```python
from build123d import *

# Parameters (mm, degrees)
SKETCH1_W           = 620
SKETCH1_H           = 130
SKETCH1_R           = 10
SKETCH1_W_2         = 18
SKETCH1_H_2         = 50
SKETCH1_W_3         = 37.615580966
SKETCH1_H_3         = 15.499548612
BOSS_EXTRUDE1_DEPTH = 18


with BuildPart() as part:
    # Sketch1 → Boss-Extrude1 (new body)
    with BuildSketch(Plane.XY):
        with Locations((310, -65)):
            Rectangle(SKETCH1_W, SKETCH1_H)
        with Locations((310, -65)):
            Circle(SKETCH1_R, mode=Mode.SUBTRACT)
        with Locations((22.856274172, -65)):
            Rectangle(SKETCH1_W_2, SKETCH1_H_2, mode=Mode.SUBTRACT)
        with Locations((310, -104.250225694)):
            Rectangle(SKETCH1_W_3, SKETCH1_H_3, mode=Mode.SUBTRACT)
        with Locations((597.143725828, -65)):
            Rectangle(SKETCH1_W_2, SKETCH1_H_2, mode=Mode.SUBTRACT)
    extrude(amount=BOSS_EXTRUDE1_DEPTH)


solid = part.part
```
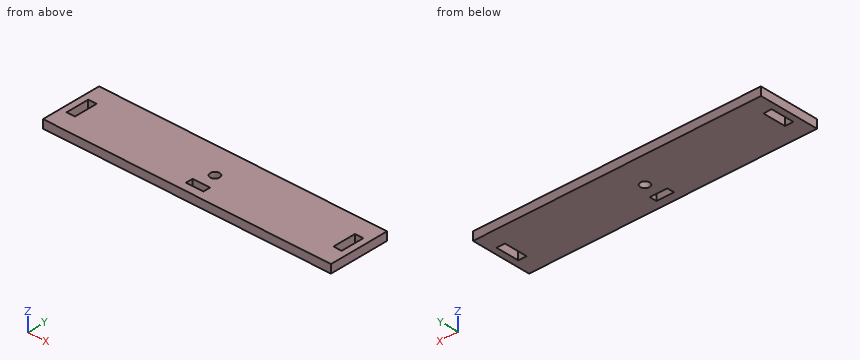
Part model, mm, in its own coordinate system. Round coordinates to 2 decimals unless told otherwise and drop trailing zeros. Loops run counter-clockwise (first coordinate to the right, second up) from the corner with the lowest first, then second, coordinate; pieces in that order, holes last. Notation, with made-up numbers: (46, -15) -> (68, -15) arc R36 ccw to (68, 21) -> close; hole circle Ø8 at (46, 6). An arc over 180 degrees is marked (long way). Use CSV: the item, a comma, the result in double quotes. Start each with the question number.
1) Cut at B-B, the plane z = 3.5. Write the cut outline in (x, y), plus the area to 3 significant figures.
2) Cut at C-C, the plane y = -65. Write the cut outline in (x, z), plus the area to 3 significant figures.
3) Cut at A-A, the plane x = 310. Write the cut outline in (y, z), plus the area to 3 significant figures.
4) Wall check: L1, parallel to Y at x = 310, z = 12.75; L2, parallel to X at y = -49, z = 2.5; L3, parallel to X at y = -101.5, z = 17. Give the ranges that are in metal, low to high. Write a range as [from, to].
5) Drop a flat-ended pin along its axis: P1, Ø5.5, axis at x = 593.5, z = 8.5, coming from the +Y side. Give the stop position or say it passes through.
Determined:
1,outline,"(0, -130) -> (620, -130) -> (620, 0) -> (0, 0) -> close; hole (13.86, -90) -> (31.86, -90) -> (31.86, -40) -> (13.86, -40) -> close; hole (291.19, -112) -> (328.81, -112) -> (328.81, -96.5) -> (291.19, -96.5) -> close; hole circle Ø20 at (310, -65); hole (588.14, -90) -> (606.14, -90) -> (606.14, -40) -> (588.14, -40) -> close"
1,area,"77,900 mm2"
2,outline,"(0, 0) -> (13.86, 0) -> (13.86, 18) -> (0, 18) -> close; (31.86, 0) -> (300, 0) -> (300, 18) -> (31.86, 18) -> close; (320, 0) -> (588.14, 0) -> (588.14, 18) -> (320, 18) -> close; (606.14, 0) -> (620, 0) -> (620, 18) -> (606.14, 18) -> close"
2,area,"10,200 mm2"
3,outline,"(-130, 0) -> (-112, 0) -> (-112, 18) -> (-130, 18) -> close; (-96.5, 0) -> (-75, 0) -> (-75, 18) -> (-96.5, 18) -> close; (-55, 0) -> (0, 0) -> (0, 18) -> (-55, 18) -> close"
3,area,"1,700 mm2"
4,L1,"y = [-130, -112], [-96.5, -75], [-55, 0]"
4,L2,"x = [0, 13.86], [31.86, 588.14], [606.14, 620]"
4,L3,"x = [0, 291.19], [328.81, 620]"
5,P1,"stops at y = 0"
